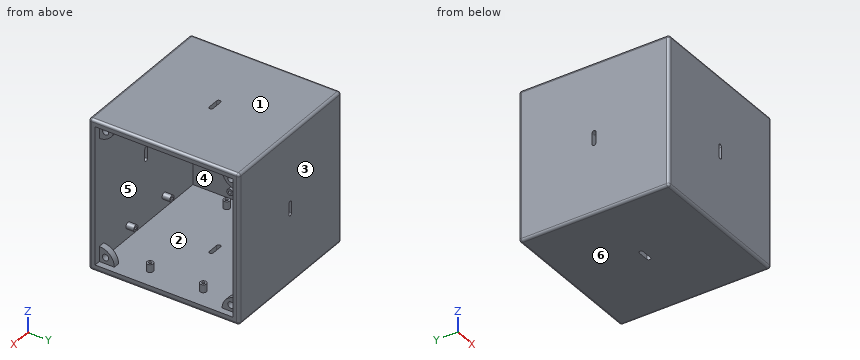
from build123d import *

# Parameters (mm, degrees)
SKETCH1_W           = 152.4
SKETCH1_H           = 152.4
BOSS_EXTRUDE1_DEPTH = 152.4
SHELL2_T            = -6.35
CUT_EXTRUDE3_DEPTH  = 6.35
CUT_EXTRUDE4_DEPTH  = 6.35
CUT_EXTRUDE5_START  = -6.35
CUT_EXTRUDE5_DEPTH  = 6.35
CUT_EXTRUDE6_DEPTH  = 6.35
SKETCH6_W           = 6.35
SKETCH6_H           = 152.4
BOSS_EXTRUDE2_DEPTH = 139.7
CUT_EXTRUDE7_DEPTH  = 6.35
SKETCH8_R           = 3.175
CUT_EXTRUDE8_DEPTH  = 6.35
SKETCH10_R          = 3.175
SKETCH10_R_2        = 1.42875
BOSS_EXTRUDE3_DEPTH = 7.9375
SKETCH11_R          = 3.175
SKETCH11_R_2        = 1.42875
BOSS_EXTRUDE4_DEPTH = 7.9375
SKETCH15_R          = 3.175
SKETCH15_R_2        = 1.42875
BOSS_EXTRUDE5_DEPTH = 7.9375
FILLET1_R           = 2.54
FILLET2_R           = 2.54


with BuildPart() as part:
    # Sketch1 → Boss-Extrude1 (new body)
    with BuildSketch(Plane(origin=(0, 0, 0), x_dir=(1, 0, 0), z_dir=(0, 1, 0))):
        Rectangle(SKETCH1_W, SKETCH1_H)
    extrude(amount=BOSS_EXTRUDE1_DEPTH)

    # Shell2
    shell2_openings = [part.faces().sort_by_distance(p)[0] for p in [
        (76.2, 76.2, 0),
    ]]
    offset(amount=SHELL2_T, openings=shell2_openings, kind=Kind.INTERSECTION)

    # Sketch2 → Cut-Extrude3 (cut)
    with BuildSketch(Plane(origin=(-69.85, 0, 0), x_dir=(0, 0, -1), z_dir=(1, 0, 0))):
        with BuildLine():
            Line((0, 76.2), (-6.498479396, 74.467072161))
            ThreePointArc((-6.498479396, 74.467072161), (-6.016790249, 74.267921368), (-5.5, 74.2))
            Line((-5.5, 74.2), (5.5, 74.2))
            ThreePointArc((5.5, 74.2), (6.016790249, 74.267921368), (6.498479396, 74.467072161))
            Line((6.498479396, 74.467072161), (0, 76.2))
        make_face()
        with BuildLine():
            Line((6.498479396, 77.932927839), (0, 76.2))
            Line((0, 76.2), (6.498479396, 74.467072161))
            ThreePointArc((6.498479396, 74.467072161), (7.5, 76.2), (6.498479396, 77.932927839))
        make_face()
        with BuildLine():
            Line((-6.498479396, 77.932927839), (0, 76.2))
            Line((0, 76.2), (6.498479396, 77.932927839))
            ThreePointArc((6.498479396, 77.932927839), (6.016790249, 78.132078632), (5.5, 78.2))
            Line((5.5, 78.2), (-5.5, 78.2))
            ThreePointArc((-5.5, 78.2), (-6.016790249, 78.132078632), (-6.498479396, 77.932927839))
        make_face()
        with BuildLine():
            ThreePointArc((-6.498479396, 77.932927839), (-7.5, 76.2), (-6.498479396, 74.467072161))
            Line((-6.498479396, 74.467072161), (0, 76.2))
            Line((0, 76.2), (-6.498479396, 77.932927839))
        make_face()
    extrude(amount=-CUT_EXTRUDE3_DEPTH, mode=Mode.SUBTRACT)

    # Sketch3 → Cut-Extrude4 (cut)
    with BuildSketch(Plane.XY.offset(-69.85)):
        with BuildLine():
            Line((-5.5, 78.2), (5.5, 78.2))
            ThreePointArc((5.5, 78.2), (7.5, 76.2), (5.5, 74.2))
            Line((5.5, 74.2), (-5.5, 74.2))
            ThreePointArc((-5.5, 74.2), (-7.5, 76.2), (-5.5, 78.2))
        make_face()
    extrude(amount=-CUT_EXTRUDE4_DEPTH, mode=Mode.SUBTRACT)

    # Sketch4 → Cut-Extrude5 (cut)
    with BuildSketch(Plane(origin=(0, 0, 69.85), x_dir=(-1, 0, 0), z_dir=(0, 0, -1)).offset(CUT_EXTRUDE5_START)):
        with BuildLine():
            Line((-5.5, 78.2), (5.5, 78.2))
            ThreePointArc((5.5, 78.2), (7.5, 76.2), (5.5, 74.2))
            Line((5.5, 74.2), (-5.5, 74.2))
            ThreePointArc((-5.5, 74.2), (-7.5, 76.2), (-5.5, 78.2))
        make_face()
    extrude(amount=CUT_EXTRUDE5_DEPTH, mode=Mode.SUBTRACT)

    # Sketch5 → Cut-Extrude6 (cut)
    with BuildSketch(Plane.XZ.offset(-146.05)):
        with BuildLine():
            Line((-2, -5.5), (-2, 5.5))
            ThreePointArc((-2, 5.5), (0, 7.5), (2, 5.5))
            Line((2, 5.5), (2, -5.5))
            ThreePointArc((2, -5.5), (0, -7.5), (-2, -5.5))
        make_face()
    cut_extrude6 = extrude(amount=-CUT_EXTRUDE6_DEPTH, mode=Mode.SUBTRACT)

    # Mirror1: Cut-Extrude6 across plane
    add(cut_extrude6.mirror(Plane.ZX.offset(76.2)), mode=Mode.SUBTRACT)

    # Sketch6 → Boss-Extrude2 (add)
    with BuildSketch(Plane.XZ.offset(-146.05)):
        with Locations((66.675, 0)):
            Rectangle(SKETCH6_W, SKETCH6_H)
    extrude(amount=BOSS_EXTRUDE2_DEPTH)

    # Sketch7 → Cut-Extrude7 (cut)
    with BuildSketch(Plane(origin=(69.85, 0, 0), x_dir=(0, 0, -1), z_dir=(1, 0, 0))):
        with BuildLine():
            Line((69.85, 21.59), (69.85, 130.81))
            ThreePointArc((69.85, 130.81), (59.073692655, 135.273692655), (54.61, 146.05))
            Line((54.61, 146.05), (-54.61, 146.05))
            ThreePointArc((-54.61, 146.05), (-59.073692655, 135.273692655), (-69.85, 130.81))
            Line((-69.85, 130.81), (-69.85, 21.59))
            ThreePointArc((-69.85, 21.59), (-59.073692655, 17.126307345), (-54.61, 6.35))
            Line((-54.61, 6.35), (54.61, 6.35))
            ThreePointArc((54.61, 6.35), (59.073692655, 17.126307345), (69.85, 21.59))
        make_face()
    extrude(amount=-CUT_EXTRUDE7_DEPTH, mode=Mode.SUBTRACT)

    # Sketch8 → Cut-Extrude8 (cut)
    with BuildSketch(Plane(origin=(69.85, 0, 0), x_dir=(0, 0, -1), z_dir=(1, 0, 0))):
        with Locations((63.5, 12.7)):
            Circle(SKETCH8_R)
        with Locations(Location((63.5, 139.7, 0), (0, 0, 180))):
            Circle(SKETCH8_R)
        with Locations((-63.5, 139.7)):
            Circle(SKETCH8_R)
        with Locations(Location((-63.5, 12.7, 0), (0, 0, 180))):
            Circle(SKETCH8_R)
    extrude(amount=-CUT_EXTRUDE8_DEPTH, mode=Mode.SUBTRACT)

    # Sketch10 → Boss-Extrude3 (add)
    # profile 1 of 4: a face of its own
    with BuildSketch(Plane(origin=(0, 0, 69.85), x_dir=(-1, 0, 0), z_dir=(0, 0, -1))):
        with Locations((-57.15, 103.1875)):
            Circle(SKETCH10_R)
        with Locations((-57.15, 103.1875)):
            Circle(SKETCH10_R_2, mode=Mode.SUBTRACT)
    # profile 2 of 4: a face of its own
    with BuildSketch(Plane(origin=(0, 0, 69.85), x_dir=(-1, 0, 0), z_dir=(0, 0, -1))):
        with Locations((-57.15, 49.2125)):
            Circle(SKETCH10_R)
        with Locations((-57.15, 49.2125)):
            Circle(SKETCH10_R_2, mode=Mode.SUBTRACT)
    # profile 3 of 4: a face of its own
    with BuildSketch(Plane(origin=(0, 0, 69.85), x_dir=(-1, 0, 0), z_dir=(0, 0, -1))):
        with Locations((57.15, 49.2125)):
            Circle(SKETCH10_R)
        with Locations((57.15, 49.2125)):
            Circle(SKETCH10_R_2, mode=Mode.SUBTRACT)
    # profile 4 of 4: a face of its own
    with BuildSketch(Plane(origin=(0, 0, 69.85), x_dir=(-1, 0, 0), z_dir=(0, 0, -1))):
        with Locations((57.15, 103.1875)):
            Circle(SKETCH10_R)
        with Locations((57.15, 103.1875)):
            Circle(SKETCH10_R_2, mode=Mode.SUBTRACT)
    boss_extrude3 = extrude(amount=BOSS_EXTRUDE3_DEPTH)

    # Mirror2: Boss-Extrude3 across plane
    add(boss_extrude3.mirror(Plane.XY))

    # Sketch11 → Boss-Extrude4 (add)
    # profile 1 of 4: a face of its own
    with BuildSketch(Plane(origin=(0, 6.35, 0), x_dir=(1, 0, 0), z_dir=(0, 1, 0))):
        with Locations(Location((-26.9875, -57.15, 0), (0, 0, 90))):
            Circle(SKETCH11_R)
        with Locations(Location((-26.9875, -57.15, 0), (0, 0, 270))):
            Circle(SKETCH11_R_2, mode=Mode.SUBTRACT)
    # profile 2 of 4: a face of its own
    with BuildSketch(Plane(origin=(0, 6.35, 0), x_dir=(1, 0, 0), z_dir=(0, 1, 0))):
        with Locations(Location((26.9875, -57.15, 0), (0, 0, 90))):
            Circle(SKETCH11_R)
        with Locations(Location((26.9875, -57.15, 0), (0, 0, 270))):
            Circle(SKETCH11_R_2, mode=Mode.SUBTRACT)
    # profile 3 of 4: a face of its own
    with BuildSketch(Plane(origin=(0, 6.35, 0), x_dir=(1, 0, 0), z_dir=(0, 1, 0))):
        with Locations(Location((26.9875, 57.15, 0), (0, 0, 90))):
            Circle(SKETCH11_R)
        with Locations(Location((26.9875, 57.15, 0), (0, 0, 270))):
            Circle(SKETCH11_R_2, mode=Mode.SUBTRACT)
    # profile 4 of 4: a face of its own
    with BuildSketch(Plane(origin=(0, 6.35, 0), x_dir=(1, 0, 0), z_dir=(0, 1, 0))):
        with Locations(Location((-26.9875, 57.15, 0), (0, 0, 90))):
            Circle(SKETCH11_R)
        with Locations(Location((-26.9875, 57.15, 0), (0, 0, 270))):
            Circle(SKETCH11_R_2, mode=Mode.SUBTRACT)
    boss_extrude4 = extrude(amount=BOSS_EXTRUDE4_DEPTH)

    # Mirror3: Boss-Extrude4 across plane
    add(boss_extrude4.mirror(Plane.ZX.offset(76.2)))

    # Sketch15 → Boss-Extrude5 (add)
    # profile 1 of 4: a face of its own
    with BuildSketch(Plane(origin=(-69.85, 0, 0), x_dir=(0, 0, -1), z_dir=(1, 0, 0))):
        with Locations((-57.15, 103.1875)):
            Circle(SKETCH15_R)
        with Locations((-57.15, 103.1875)):
            Circle(SKETCH15_R_2, mode=Mode.SUBTRACT)
    # profile 2 of 4: a face of its own
    with BuildSketch(Plane(origin=(-69.85, 0, 0), x_dir=(0, 0, -1), z_dir=(1, 0, 0))):
        with Locations((-57.15, 49.2125)):
            Circle(SKETCH15_R)
        with Locations((-57.15, 49.2125)):
            Circle(SKETCH15_R_2, mode=Mode.SUBTRACT)
    # profile 3 of 4: a face of its own
    with BuildSketch(Plane(origin=(-69.85, 0, 0), x_dir=(0, 0, -1), z_dir=(1, 0, 0))):
        with Locations((57.15, 49.2125)):
            Circle(SKETCH15_R)
        with Locations((57.15, 49.2125)):
            Circle(SKETCH15_R_2, mode=Mode.SUBTRACT)
    # profile 4 of 4: a face of its own
    with BuildSketch(Plane(origin=(-69.85, 0, 0), x_dir=(0, 0, -1), z_dir=(1, 0, 0))):
        with Locations((57.15, 103.1875)):
            Circle(SKETCH15_R)
        with Locations((57.15, 103.1875)):
            Circle(SKETCH15_R_2, mode=Mode.SUBTRACT)
    extrude(amount=BOSS_EXTRUDE5_DEPTH)

    # Fillet1
    fillet1_edges = [part.edges().sort_by_distance(p)[0] for p in [
        (76.2, 76.2, 76.2),
        (-76.2, 76.2, 76.2),
        (-76.2, 76.2, -76.2),
        (76.2, 76.2, -76.2),
    ]]
    fillet(fillet1_edges, radius=FILLET1_R)

    # Fillet2
    fillet2_edges = [part.edges().sort_by_distance(p)[0] for p in [
        (76.2, 0, 0),
        (76.2, 152.4, 0),
        (0, 0, 76.2),
        (-76.2, 0, 0),
        (0, 0, -76.2),
        (75.456051224, 0, -75.456051224),
        (-75.456051224, 0, -75.456051224),
        (-75.456051224, 0, 75.456051224),
        (75.456051224, 0, 75.456051224),
        (0, 152.4, 76.2),
        (0, 152.4, -76.2),
        (-76.2, 152.4, 0),
        (75.456051224, 152.4, -75.456051224),
        (-75.456051224, 152.4, -75.456051224),
        (-75.456051224, 152.4, 75.456051224),
        (75.456051224, 152.4, 75.456051224),
    ]]
    fillet(fillet2_edges, radius=FILLET2_R)


solid = part.part
Build history of the part. All positions in model axes, mm. Face numbers are marked on the shaded views. A direction names the side the tool comes from. Round coordinates to 2 decimals unless told otherwise and drop trailing zeros. Loops run counter-clockwise (first coordinate to the right, second up) from the corner with the lowest first, then second, coordinate; pieces in that order, holes last. Notation, with made-up numbers: (58.25, 75.25) -> (71.25, 75.25) arc R26 ccw to (71.25, 93.25) -> close; hole circle Ø2 at (-29, -13.75). An arc over 180 degrees is marked (long way). Use CSV: the item, a comma, the result in double quotes. Start each with the question number.
Q1. Saw through at D-D on y = 112. Give the cut face in (x, z), and give its area (3 significant figures).
Q2. Flat gauge pins, fed straight in: pin 1 Ø6 at (y, z) = (77, -35.5) entering from +X; pin 2 Ø4.5 at (y, z) = (14, 61.5) entering from +X; pin 3 Ø3 at (y, z) = (49.5, 58.5) entering from +X. Where does each tip first touch, or does it go through?
Q3. Saw through at C-C on z = -22. Give the cut face in (x, y).
Q4. Saw through at B-B on x = 67.5. Give the cut face in (y, z) (3 decimals).
Q5. Which spindle directions (+Z, -Z, +X, -X, +Y, -Y) get a long thin tool onto all of the face, cutting with end or side? Do the marked faces 1 and 2. Say none if no direction does.
Q6. Saw through at A-A on x = -49.5. Give the cut face in (y, z).
Q7. Mould opens along Z. For the marked faces 3, 4, 5 and 6 say: +Z half, -Z half, draft (parallel to the pull), parting line (faces both ways), or undercut.
Q8. Drill centre lines: L1, parallel to X at y = 142, z = 57; L2, parallel to Y at x = -57, z = 66; L3, parallel to Y at x = 23, z = 58.5. Where is each one in solid material? Low to high.
Solutions:
1,outline,"(-76.2, -73.66) arc R2.54 ccw to (-73.66, -76.2) -> (73.66, -76.2) arc R2.54 ccw to (76.2, -73.66) -> (76.2, -69.85) -> (-69.85, -69.85) -> (-69.85, 69.85) -> (76.2, 69.85) -> (76.2, 73.66) arc R2.54 ccw to (73.66, 76.2) -> (-73.66, 76.2) arc R2.54 ccw to (-76.2, 73.66) -> close"
1,area,"2,820 mm^2"
2,pin 1,"stops at x = -69.85"
2,pin 2,"stops at x = 69.85"
2,pin 3,"stops at x = -61.91"
3,outline,"(-76.2, 2.54) arc R2.54 ccw to (-73.66, 0) -> (73.66, 0) arc R2.54 ccw to (76.2, 2.54) -> (76.2, 6.35) -> (-69.85, 6.35) -> (-69.85, 146.05) -> (76.2, 146.05) -> (76.2, 149.86) arc R2.54 ccw to (73.66, 152.4) -> (-73.66, 152.4) arc R2.54 ccw to (-76.2, 149.86) -> close"
4,outline,"(0, -73.66) arc R2.54 ccw to (2.54, -76.2) -> (149.86, -76.2) arc R2.54 ccw to (152.4, -73.66) -> (152.4, 73.66) arc R2.54 ccw to (149.86, 76.2) -> (2.54, 76.2) arc R2.54 ccw to (0, 73.66) -> close; hole (6.35, -54.61) arc R15.24 cw to (21.59, -69.85) -> (130.81, -69.85) arc R15.24 cw to (146.05, -54.61) -> (146.05, 54.61) arc R15.24 cw to (130.81, 69.85) -> (21.59, 69.85) arc R15.24 cw to (6.35, 54.61) -> close; hole circle Ø6.35 at (12.7, -63.5); hole circle Ø6.35 at (12.7, 63.5); hole circle Ø6.35 at (139.7, -63.5); hole circle Ø6.35 at (139.7, 63.5)"
5,face 1,"+Z, +X, -X, +Y, -Y"
5,face 2,"none"
6,outline,"(0, -73.66) arc R2.54 ccw to (2.54, -76.2) -> (149.86, -76.2) arc R2.54 ccw to (152.4, -73.66) -> (152.4, 73.66) arc R2.54 ccw to (149.86, 76.2) -> (2.54, 76.2) arc R2.54 ccw to (0, 73.66) -> close; hole (6.35, -69.85) -> (146.05, -69.85) -> (146.05, 69.85) -> (6.35, 69.85) -> close"
7,face 3,"draft"
7,face 4,"undercut"
7,face 5,"undercut"
7,face 6,"-Z half"
8,L1,"x = -76.2 to -69.85, -30.16 to -28.41, -25.57 to -23.82, 23.82 to 25.57, 28.41 to 30.16, 63.5 to 69.85"
8,L2,"y = 0 to 6.35, 46.04 to 47.79, 50.63 to 52.38, 100.02 to 101.77, 104.61 to 106.36, 146.05 to 152.4"
8,L3,"y = 0 to 6.35, 146.05 to 152.4"
